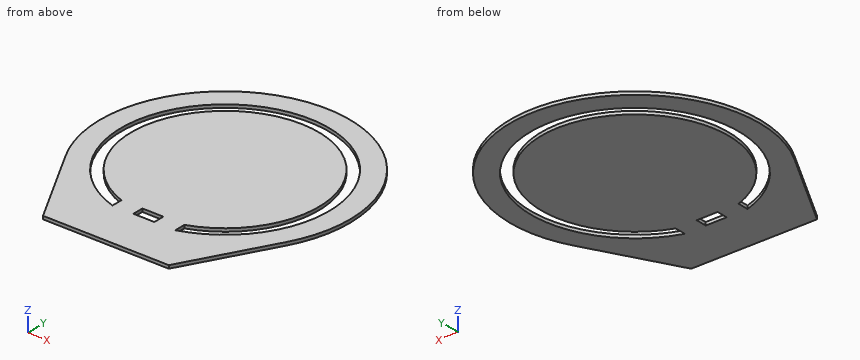
from build123d import *

# Parameters (mm, degrees)
BOSS_EXTRUDE1_DEPTH = 0.75438


with BuildPart() as part:
    # Sketch1 → Boss-Extrude1 (new body)
    with BuildSketch(Plane.XY):
        with BuildLine():
            Line((-26.292884648, -14.44590658), (-15, -35))
            Line((-15, -35), (-7.5, -35))
            Line((-7.5, -35), (15, -35))
            Line((15, -35), (26.292884648, -14.44590658))
            ThreePointArc((26.292884648, -14.44590658), (0, 30), (-26.292884648, -14.44590658))
        make_face()
        Polygon((2.5, -23.848480035), (-2.5, -23.848480035), (-2.5, -22.360679775), (-2.5, -21.213203436), (2.5, -21.213203436), (2.5, -22.360679775), align=None, mode=Mode.SUBTRACT)
        with BuildLine():
            Line((-7.5, -21.213203436), (-7.5, -23.848480035))
            ThreePointArc((-7.5, -23.848480035), (0, 25), (7.5, -23.848480035))
            Line((7.5, -23.848480035), (7.5, -21.213203436))
            ThreePointArc((7.5, -21.213203436), (0, 22.5), (-7.5, -21.213203436))
        make_face(mode=Mode.SUBTRACT)
    extrude(amount=BOSS_EXTRUDE1_DEPTH)


solid = part.part
Input: part model. Units: mm. Frame: model coordinates. Round coordinates to 2 decimals unless told otherwise and drop trailing zeros. Order: outer loops, then holes, each group sorted by start corner. A loop starts at its lowest first (then second) coordinate and runs counter-clockwise, first axis right, second up.
1. Cut plane A-A, the plane y = 0. Output: boundary loops of the cut face in (x, z), then the cut area to 3 significant figures.
The answers:
outline: (-30, 0) - (-25, 0) - (-25, 0.75) - (-30, 0.75) - close; (-22.5, 0) - (22.5, 0) - (22.5, 0.75) - (-22.5, 0.75) - close; (25, 0) - (30, 0) - (30, 0.75) - (25, 0.75) - close
area: 41.5 mm2
2. Cut plane C-C, the plane z = 0.3. Output: boundary loops of the cut face in (x, y).
The answers:
outline: (-26.29, -14.45) - (-15, -35) - (15, -35) - (26.29, -14.45) arc R30 ccw (long way) to start; hole (-7.5, -23.85) - (-7.5, -21.21) arc R22.5 cw (long way) to (7.5, -21.21) - (7.5, -23.85) arc R25 ccw (long way) to start; hole (-2.5, -23.85) - (2.5, -23.85) - (2.5, -21.21) - (-2.5, -21.21) - close
3. Cut plane B-B, the plane x = 0. Output: boundary loops of the cut face in (y, z).
The answers:
outline: (-35, 0) - (-23.85, 0) - (-23.85, 0.75) - (-35, 0.75) - close; (-21.21, 0) - (22.5, 0) - (22.5, 0.75) - (-21.21, 0.75) - close; (25, 0) - (30, 0) - (30, 0.75) - (25, 0.75) - close
4. Material intervals for line 1 (X direction, y = 0, z = 0.3); line 2 (Y direction, x = 0, z = 0.55); line 3 (X direction, y = -7.5, z = 0.1), sorted ascending.
The answers:
line 1: x = -30 to -25, -22.5 to 22.5, 25 to 30
line 2: y = -35 to -23.85, -21.21 to 22.5, 25 to 30
line 3: x = -29.05 to -23.85, -21.21 to 21.21, 23.85 to 29.05
